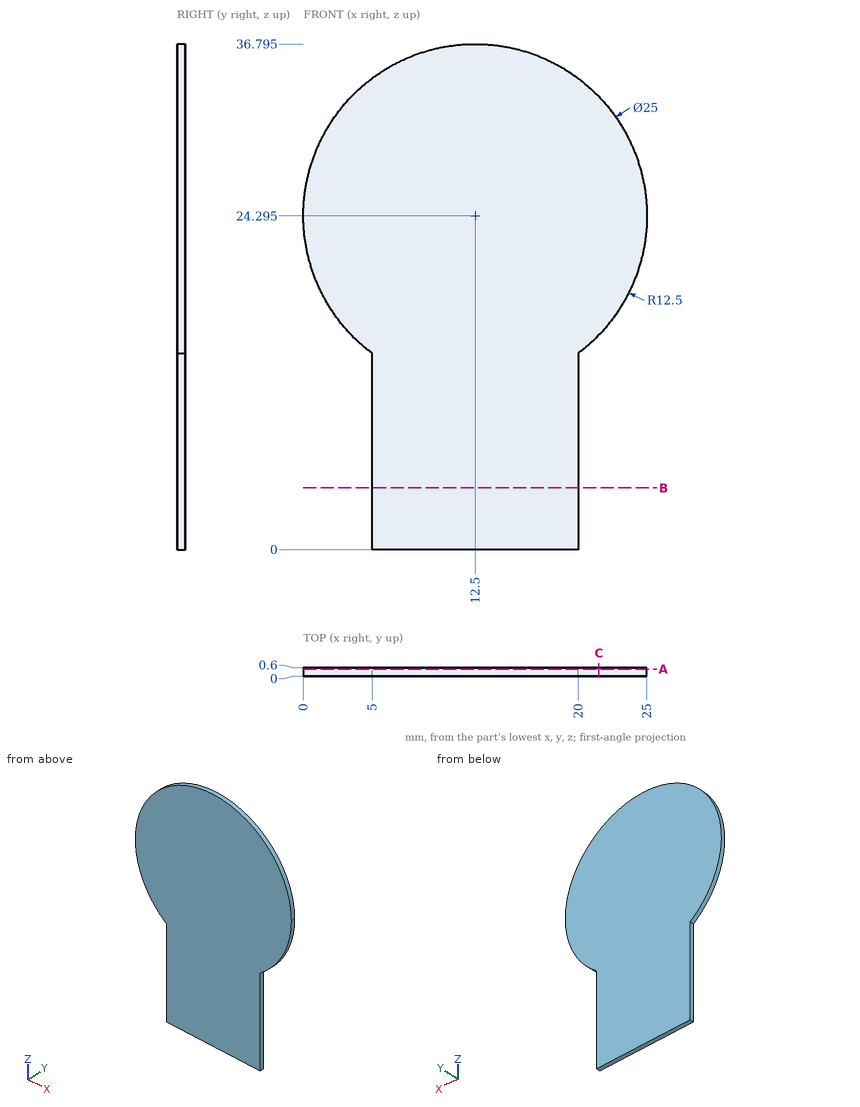
Could you check a few things on this drawing? It's one solid part, dimensions in mm from its lowest x, y, z. Round coordinates to 2 decimals unless told otherwise and drop trailing zeros. Loops run counter-clockwise (first coordinate to the right, second up) from the corner with the lowest first, then second, coordinate; pieces in that order, holes last. Notation, with made-up numbers: M 89,-7 L 142,-7 A28 ccw 142,20 Z; hole C 39,21.25 d7. An arc over 180 degrees is marked long. Write each question's results on one line, items separated by ' | '. Start each with the question number.
(1) If I drill on probe 1 along X at (y, z) = (0.1, 9.5); probe 2 along Z at (x, y) = (3.75, 0.45); probe 3 along X at (y, z) = (0.45, 17), over which ranges is the centre line in solid material (lowest first)? Write a range as from..to.
(2) I want a section at A-A (y = 0.5). Please give me the cut outline in (x, z) (1 decimal).
(3) I want a section at C-C (x = 21.5). Please give me the cut outline in (y, z), then the cut area to 3 significant figures.
(4) I want a section at B-B (z = 4.5). Please give me the cut outline in (x, y).
Solved:
1) probe 1: x = 5..20 | probe 2: z = 15.37..33.22 | probe 3: x = 2.35..22.65
2) outline: M 5,0 L 20,0 L 20,14.3 A12.5 ccw long 5,14.3 Z
3) outline: M 0,15.62 L 0.6,15.62 L 0.6,32.97 L 0,32.97 Z | area: 10.4 mm²
4) outline: M 5,0 L 20,0 L 20,0.6 L 5,0.6 Z
